Geometry: final body of the model. Coordinates: model frame, mm. A direction names the side the tool comes from. Give positions to 0.01 mm unless a question says otherwise; leave off trailing zeros. Loops run counter-clockwise (first coordinate to the right, second up) from the corner with the lowest first, then second, coordinate; pieces in that order, holes last. Notation, with made-up numbers: (-28, 54.5) -> (27, 54.5) arc R33 ccw to (27, 90.5) -> close; hole circle Ø8 at (33, 43.5). An arc over 180 degrees is marked (long way). One line per item, written item: value. Start each with the question number.
from build123d import *

# Parameters (mm, degrees)
SKETCH1_R             = 3.75
BOSS_EXTRUDE1_DEPTH   = 27
M4_TAPPED_HOLE1_D     = 3.3
M4_TAPPED_HOLE1_DEPTH = 5
M4_TAPPED_HOLE1_TIP   = 0.991420021
M4_TAPPED_HOLE2_D     = 3.3
M4_TAPPED_HOLE2_DEPTH = 7.1
M4_TAPPED_HOLE2_TIP   = 0.991420021
SCALE1_SCALE          = 1.013


with BuildPart() as part:
    # Sketch1 → Boss-Extrude1 (new body)
    with BuildSketch(Plane.XY):
        Circle(SKETCH1_R)
    extrude(amount=BOSS_EXTRUDE1_DEPTH)

    # M4 Tapped Hole1
    with Locations(Plane.XY.offset(27)):
        with Locations((0, 0)):
            Hole(M4_TAPPED_HOLE1_D / 2, depth=M4_TAPPED_HOLE1_DEPTH)
            with Locations((0, 0, -(M4_TAPPED_HOLE1_DEPTH + M4_TAPPED_HOLE1_TIP / 2))):  # 118° drill point
                Cone(0, M4_TAPPED_HOLE1_D / 2, M4_TAPPED_HOLE1_TIP, mode=Mode.SUBTRACT)

    # M4 Tapped Hole2
    with Locations(Plane(origin=(0, 0, 0), x_dir=(-1, 0, 0), z_dir=(0, 0, -1))):
        with Locations((0, 0)):
            Hole(M4_TAPPED_HOLE2_D / 2, depth=M4_TAPPED_HOLE2_DEPTH)
            with Locations((0, 0, -(M4_TAPPED_HOLE2_DEPTH + M4_TAPPED_HOLE2_TIP / 2))):  # 118° drill point
                Cone(0, M4_TAPPED_HOLE2_D / 2, M4_TAPPED_HOLE2_TIP, mode=Mode.SUBTRACT)


with BuildPart() as part_1:
    # Scale1: scaled about (0, 0, 13.618001469)
    add(part.part.scale(SCALE1_SCALE).moved(Location((0, 0, -0.177034019))))


solid = part_1.part
Item 1: Section C-C, the plane x = 2.5. Output: boundary loops of the cut face in (y, z), then the cut area to 3 significant figures.
Item 2: Pin query (flat end, axial travel): pin 1 (3 mm diameter, centred on x = 0, y = 0, fed in from +Z); pin 2 (1.5 mm diameter, centred on y = 3, z = 8.5, fed in from -X). Return the tip coordinate at first contact, or that it passes through.
Item 3: Mould query, pull axis X, two halves, no side actions, for faces 1 (the face through (-0.277, 0.087, 7.845)), 2 (the face through (2, -1, -0.177)), 3 (the face through (-3.015, -2.311, 13.307)). Classes: pulls with the +X half, pulls with the -X half, needs draft (parallel to the pull), parting line crosses it, or undercut.
Item 4: Section D-D, the plane y = -3. Output: boundary loops of the cut face in (x, z).
Item 5: Section A-A, the plane z = 5. Output: boundary loops of the cut face in (x, y), then the cut area to 3 significant figures.
Item 6: Ray query, line 1 along Y through (x, z) = (0, 3); line 2 along X through (y, z) = (2, 22.5); line 3 along X through (y, z) = (-2.25, 3.75). Return the intervals inside material, ascending. Write a range as [from, to].
Item 7: Section B-B, the plane z = 15.5. Output: boundary loops of the cut face in (x, y).
Item 8: Access query for faces 4 (the face through (-0.362, -1.632, 3.469)), 5 (the face through (0.362, -1.632, 24.606)), 6 (the face through (2, -1, 27.174)). Directions: +Z, -Z, +X, -X, +Y, -Y. A direction counts if a zero-diameter tool reaches every point of the face in a straight line with its end or side. Return the directions, or none.
Geometry check:
1. outline: (-2.86, -0.18) -> (2.86, -0.18) -> (2.86, 27.17) -> (-2.86, 27.17) -> close
1. area: 156 mm2
2. pin 1: stops at z = 22.01
2. pin 2: stops at x = -3.06
3. face 1: undercut
3. face 2: needs draft
3. face 3: parting line crosses it
4. outline: (-2.33, -0.18) -> (2.33, -0.18) -> (2.33, 27.17) -> (-2.33, 27.17) -> close
5. outline: circle Ø7.6 at (0, 0); hole circle Ø3.34 at (0, 0)
5. area: 36.6 mm2
6. line 1: y = [-3.8, -1.67], [1.67, 3.8]
6. line 2: x = [-3.23, 3.23]
6. line 3: x = [-3.06, 3.06]
7. outline: circle Ø7.6 at (0, 0)
8. face 4: -Z
8. face 5: +Z
8. face 6: +Z, +X, -X, +Y, -Y
